```python
from build123d import *

# Parameters (mm, degrees)
F0_W     = 100
F0_H     = 280
F1_DEPTH = 20
F3_DEPTH = 20
F4_W     = 20
F4_H     = 20
F5_DEPTH = 20


# Not quite as in the source:
# - a feature names something its author has since deleted; it is built from what else it names


with BuildPart() as f1:
    # F0 (on Right) → F1 (new body)
    with BuildSketch(Plane.YZ):
        Rectangle(F0_W, F0_H)
    extrude(amount=F1_DEPTH)

    # F2 (on face) → F3 (cut, through all)
    with BuildSketch(Plane.YZ.offset(20)):
        with BuildLine():
            ThreePointArc((-30, 140), (12.7200187266, 132.2533832709), (50, 110))
            Line((50, 110), (50, 140))
            Line((50, 140), (-30, 140))
        make_face()
    extrude(amount=-F3_DEPTH, mode=Mode.SUBTRACT)

    # F4 (on face) → F5 (cut, through all)
    with BuildSketch(Plane(origin=(0, 0, 0), x_dir=(0, -1, 0), z_dir=(-1, 0, 0))):
        with Locations((40, -130)):
            Rectangle(F4_W, F4_H)
        with Locations((40, -90)):
            Rectangle(F4_W, F4_H)
        with Locations((40, -50)):
            Rectangle(F4_W, F4_H)
        with Locations((40, -10)):
            Rectangle(F4_W, F4_H)
        with Locations((40, 30)):
            Rectangle(F4_W, F4_H)
        with Locations((40, 70)):
            Rectangle(F4_W, F4_H)
        with Locations((40, 110)):
            Rectangle(F4_W, F4_H)
    extrude(amount=-F5_DEPTH, mode=Mode.SUBTRACT)


solid = f1.part
```
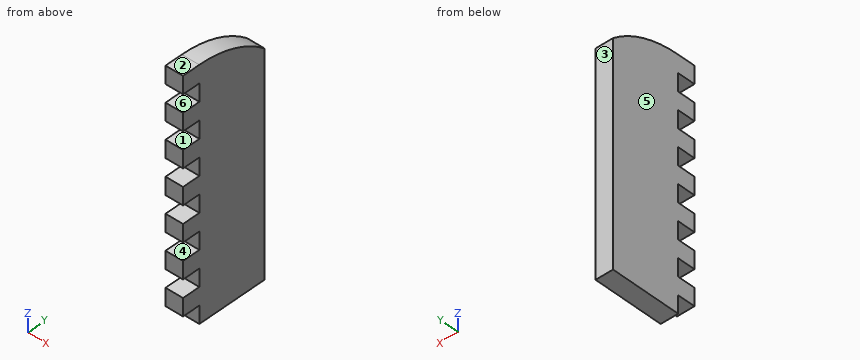
Here's how the part is built. I have some questions about the finished solid (model axes, mm). Face numbers are marked on the shaded views. A direction names the side the tool comes from. Coordinates: 2 decimals unless noted, no trailing zeros. Order: outer loops, then holes, each group sorted by start corner. A loop starts at its lowest first (then second) coordinate and runs counter-clockwise, first axis right, second up. Notation, with made-up numbers: (-3.75, 23) - (39.25, 23) arc R24 ccw to (39.25, 41) - close; hole circle Ø8 at (71.5, 39.25). An arc over 180 degrees is marked (long way). One line per question, with ' | ' between items. Start each with the question number.
1. Which directions (+Z, -Z, +X, -X, +Y, -Y) give clear straight access to the entire face, cutting with the end or side of a thin tool? Please do the marked faces 5 and 6.
2. If we section it at B-B (z = 68): Write out the boundary of the cut face in (x, y).
3. If we mould it in two halves opening along Z, with no side actions, what happens to the marked faces 1, 2, 3 and 4? For each: released by +Z, released by -Z, zero draft, split by the parting line, or undercut.
4. Please list where these lines run through material, in increasing order: line 1 along Y through (x, z) = (8, 61.5); line 2 along Z through (x, y) = (7.25, -21.5); line 3 along Y through (x, z) = (1, 126). Write a range as [from, to].
5. I'm going to push flat-ended pins straight in: pin 1 Ø10 at (x, y) = (10, -39.5) entering from -Z; pin 2 Ø10 at (x, z) = (14, -8) entering from -Y; pin 3 Ø4 at (x, y) = (15.5, 39.5) entering from +Z. Where does each tip first touch, or does it pass through?
Model answer:
1) face 5: +Z, -Z, -X, +Y, -Y | face 6: +X, -X, -Y
2) outline: (0, -30) - (20, -30) - (20, 50) - (0, 50) - close
3) face 1: undercut | face 2: released by +Z | face 3: zero draft | face 4: undercut
4) line 1: y = [-30, 50] | line 2: z = [-140, 139.7] | line 3: y = [-50, 26.66]
5) pin 1: stops at z = -120 | pin 2: stops at y = -30 | pin 3: stops at z = 119.56
